Source: CAD feature listing. Evaluate the final solid. Frame: model axes, mm. Face numbers are marked on the shaded views. Round coordinates to 2 decimals unless told otherwise and drop trailing zeros. Order: outer loops, then holes, each group sorted by start corner. A loop starts at its lowest first (then second) coordinate and runs counter-clockwise, first axis right, second up. Notation, with made-up numbers: (47, 12.5) - (62, 12.5) arc R32 cw to (62, 45.5) - close; hole circle Ø6 at (-35.75, 74.25). An arc over 180 degrees is marked (long way). Use one line per item in the form item = value. Start each with the question number.
Q1. Cut plane B-B, the plane y = 10.5. Return the cut outline in (x, z).
Q2. Pin query (flat end, axial travel): pin 1 Ø3 at (x, z) = (7.5, 1.5) entering from -Y; pin 2 Ø1.5 at (y, z) = (4.5, -2.5) entering from -X; pin 3 Ø2 at (y, z) = (9, 8) entering from +X; pin 4 Ø5 at (y, z) = (10, 6.5) entering from +X. Return the tip coordinate at first contact, or that it passes through.
Q3. Draft query along Z for the marked faces 1, 2, 3 and 4. Return one class per face: released by +Z, released by -Z, zero draft, split by the parting line, or undercut.
Q4. Cut plane A-A, the plane y = 4. Return the cut outline in (x, z).
Q5. Ray query, line 1 (X direction, y = 5.75, z = -1.5); line 2 (X direction, y = 11.5, z = 10.25); line 3 (X direction, y = 4.5, z = -0.75). Return the intervals inside material, ascending. Write a range as [from, to].
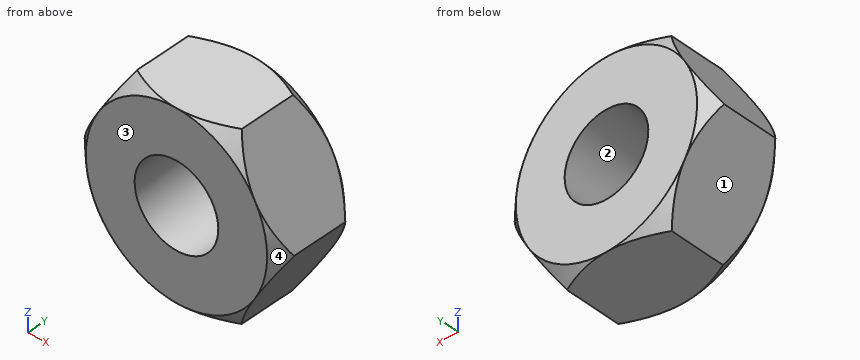
from build123d import *

# Parameters (mm, degrees)
BOSS_EXTRUDE1_DEPTH = 12
SKETCH3_R           = 6
CUT_EXTRUDE1_DEPTH  = 24.202011407
SKETCH6_OUTSIDE_W   = 88.724
SKETCH6_OUTSIDE_H   = 84.702
SKETCH6_OUTSIDE_R   = 13
CUT_EXTRUDE3_DEPTH  = 24.202011407
CUT_EXTRUDE3_DRAFT  = -45
SKETCH7_OUTSIDE_W   = 88.724
SKETCH7_OUTSIDE_H   = 84.702
SKETCH7_OUTSIDE_R   = 13
CUT_EXTRUDE4_DEPTH  = 24.202011407
CUT_EXTRUDE4_DRAFT  = -45


with BuildPart() as part:
    # Sketch2 → Boss-Extrude1 (new body)
    with BuildSketch(Plane(origin=(0, 0, 0), x_dir=(1, 0, 0), z_dir=(0, 1, 0))):
        Polygon((-15.011106999, 0), (-7.505553499, -13), (7.505553499, -13), (15.011106999, 0), (7.505553499, 13), (-7.505553499, 13), align=None)
    extrude(amount=BOSS_EXTRUDE1_DEPTH)

    # Sketch3 → Cut-Extrude1 (cut, through all)
    with BuildSketch(Plane(origin=(0, 12, 0), x_dir=(1, 0, 0), z_dir=(0, 1, 0))):
        with Locations(Location((0, 0, 0), (0, 0, 270))):
            Circle(SKETCH3_R)
    extrude(amount=-CUT_EXTRUDE1_DEPTH, mode=Mode.SUBTRACT)


with BuildPart() as cut_extrude3_tool:
    # Sketch6 outside → Cut-Extrude3 (with draft: the straight prism first)
    with BuildSketch(Plane(origin=(0, 12, 0), x_dir=(1, 0, 0), z_dir=(0, 1, 0))):
        Rectangle(SKETCH6_OUTSIDE_W, SKETCH6_OUTSIDE_H)
        Circle(SKETCH6_OUTSIDE_R, mode=Mode.SUBTRACT)
    extrude(amount=-CUT_EXTRUDE3_DEPTH)
    # Cut-Extrude3: the draft: its side faces are tilted about the plane it starts from
    cut_extrude3_sides = [cut_extrude3_tool.faces().sort_by_distance(p)[0] for p in [
        (0, -0.101005704, 42.351),
        (44.362, -0.101005704, 0),
        (0, -0.101005704, -42.351),
        (-44.362, -0.101005704, 0),
        (-13, -0.101005704, 0),
    ]]
    draft(cut_extrude3_sides, Plane(origin=(0, 12, 0), x_dir=(1, 0, 0), z_dir=(0, 1, 0)), CUT_EXTRUDE3_DRAFT)


with BuildPart() as part_1:
    add(part.part)

    # Cut-Extrude3: cut by cut_extrude3_tool
    add(cut_extrude3_tool.part, mode=Mode.SUBTRACT)


with BuildPart() as cut_extrude4_tool:
    # Sketch7 outside → Cut-Extrude4 (with draft: the straight prism first)
    with BuildSketch(Plane.XZ):
        Rectangle(SKETCH7_OUTSIDE_W, SKETCH7_OUTSIDE_H)
        Circle(SKETCH7_OUTSIDE_R, mode=Mode.SUBTRACT)
    extrude(amount=-CUT_EXTRUDE4_DEPTH)
    # Cut-Extrude4: the draft: its side faces are tilted about the plane it starts from
    cut_extrude4_sides = [cut_extrude4_tool.faces().sort_by_distance(p)[0] for p in [
        (0, 12.101005704, -42.351),
        (44.362, 12.101005704, 0),
        (0, 12.101005704, 42.351),
        (-44.362, 12.101005704, 0),
        (-13, 12.101005704, 0),
    ]]
    draft(cut_extrude4_sides, Plane.XZ, CUT_EXTRUDE4_DRAFT)


with BuildPart() as part_2:
    add(part_1.part)

    # Cut-Extrude4: cut by cut_extrude4_tool
    add(cut_extrude4_tool.part, mode=Mode.SUBTRACT)


solid = part_2.part
Completed:
q1.outline = (-14.47, -0.94) - (-8.05, -12.06) arc R14.5 ccw to (-6.42, -13) - (6.42, -13) arc R14.5 ccw to (8.05, -12.06) - (14.47, -0.94) arc R14.5 ccw to (14.47, 0.94) - (8.05, 12.06) arc R14.5 ccw to (6.42, 13) - (-6.42, 13) arc R14.5 ccw to (-8.05, 12.06) - (-14.47, 0.94) arc R14.5 ccw to start; hole circle Ø12 at (0, 0)
q2.pin_1 = 0
q2.pin_2 = -14
q2.pin_3 = 10.97
q2.pin_4 = 12.7
q3.face_1 = released by -Z
q3.face_2 = undercut
q3.face_3 = zero draft
q3.face_4 = split by the parting line
q4.outline = (-15.01, 0) - (-7.51, -13) - (7.51, -13) - (15.01, 0) - (7.51, 13) - (-7.51, 13) - close; hole circle Ø12 at (0, 0)
q5.line_1 = [-14.15, -5.81], [5.81, 14.15]
q5.line_2 = [-8.79, 8.79]
q5.line_3 = [-14.58, -5.95], [5.95, 14.58]
